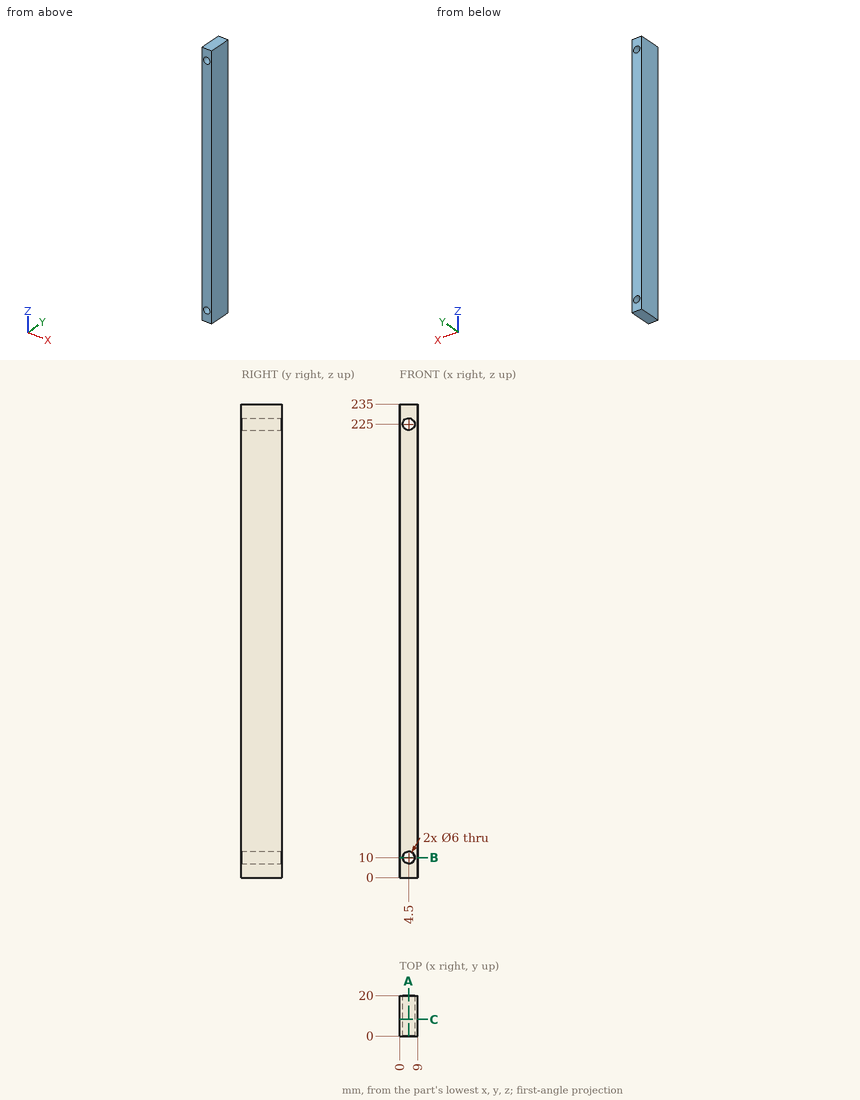
Part print with two shaded views. Sizes in mm from the minimum x, y, z corner. Round coordinates to 2 decimals unless told otherwise and drop trailing zeros. Order: outer loops, then holes, each group sorted by start corner. A loop starts at its lowest first (then second) coordinate and runs counter-clockwise, first axis right, second up. Notation, with made-up numbers: (-20.5, 19) - (17.5, 19) arc R25 ccw to (17.5, 35) - close; hole circle Ø2 at (14.5, 40.5). An arc over 180 degrees is marked (long way). Answer in a Markdown table with one row per item. Add a question column.
(1) Band-saw the part on C-C on y = 8.25. List the corners of the cut face in (x, z), and give its area (3 significant figures).
(2) Band-saw the part on B-B on z = 10. List the corners of the cut face in (x, y).
(3) Probe L1, parallel to Z at x = 4.5, y = 12.5; L2, parallel to X at y = 13, z = 10; L3, parallel to Z at x = 7.25, y = 8.25. List the from-to ranges inside material, lowest first. Write a range as [from, to].
(4) Band-saw the part on A-A on x = 4.5. List the corners of the cut face in (y, z).
Data:
| question | item | result |
|---|---|---|
| 1 | outline | (0, 0) - (9, 0) - (9, 235) - (0, 235) - close; hole circle Ø6 at (4.5, 10); hole circle Ø6 at (4.5, 225) |
| 1 | area | 2,060 mm^2 |
| 2 | outline | (0, 0) - (1.5, 0) - (1.5, 20) - (0, 20) - close; (7.5, 0) - (9, 0) - (9, 20) - (7.5, 20) - close |
| 3 | L1 | z = [0, 7], [13, 222], [228, 235] |
| 3 | L2 | x = [0, 1.5], [7.5, 9] |
| 3 | L3 | z = [0, 8.8], [11.2, 223.8], [226.2, 235] |
| 4 | outline | (0, 0) - (20, 0) - (20, 7) - (0, 7) - close; (0, 13) - (20, 13) - (20, 222) - (0, 222) - close; (0, 228) - (20, 228) - (20, 235) - (0, 235) - close |
